Here's how the part is built. I have some questions about the finished solid (model axes, mm). A direction names the side the tool comes from. Round coordinates to 2 decimals unless told otherwise and drop trailing zeros. Write each loop counter-clockwise with the first axis right and the second up, starting at its lowest first coordinate (ties: lowest second). Pieces come first, ordered by that corner, then holes. Notation, with made-up numbers: (28, 58.25) - (83, 58.25) arc R5 ccw to (83, 64.25) - close; hole circle Ø1 at (-16.5, -35). An arc over 180 degrees is marked (long way). Write item = value, one per line. Start each with the question number.
Item 1: If we section it at A-A (z = 0): Please give me the cut outline in (x, y) (1 decimal).
Item 2: If I drill on line 1 along Y through (x, z) = (8, 0); line 2 along X through (y, z) = (12, -8.5) (3 decimals); line 3 along Y through (x, z) = (16.5, 7), over which ranges is the centre line in solid material (lowest first)? Write a range as [from, to].
Item 3: Which directions (+Z, -Z, +X, -X, +Y, -Y) give clear straight access to the entire face, cutting with the end or side of a thin tool? Please do faces 1 (the face through (13.148, 0.628, 14.274)), 2 (the face through (-3.175, -8, -8)).
Item 4: If we section it at C-C (x = 9.5): Please give me the cut outline in (y, z) (1 decimal), and give its area (3 significant figures).
Item 5: Thinking about a two-plate mould opening in Y: for faces 3 (the face through (29.845, -8, -8)), 4 (the face through (13.566, 8.406, -5.36)), 5 (the face through (-2.209, -10.626, 13.858)), which applies, pulls with the +Y half, pulls with the -Y half, needs draft (parallel to the pull), parting line crosses it, or undercut?
Item 6: For P1, Ø8, axis at x = 25, z = 8.5, coming from the -Y side; P2, Ø5, axis at x = 3.5, z = -11.5, coming from the +Y side; P3, Ø5, axis at x = 14.5, y = 7.5, coming from the -Z side; P4, Ø18, axis at y = 0, z = 0, coming from the -X side (3 decimals), each with a flat end and sliding along its axis, tell me the tip position at first contact or that it passes through.
```python
from build123d import *

# Parameters (mm, degrees)
SKETCH1_R            = 14.2875
SKETCH1_R_2          = 9.9695
BOSS_EXTRUDE1_DEPTH  = 26.67
SKETCH2_R            = 17.4625
SKETCH2_R_2          = 9.9695
BOSS_EXTRUDE2_DEPTH  = 3.175
FILLET1_R            = 1.27
FILLET1_OF_MIRROR1_R = 1.27


with BuildPart() as part:
    # Sketch1 → Boss-Extrude1 (new body)
    with BuildSketch(Plane(origin=(0, 0, 0), x_dir=(0, 0, -1), z_dir=(1, 0, 0))):
        Circle(SKETCH1_R)
        Circle(SKETCH1_R_2, mode=Mode.SUBTRACT)
    extrude(amount=BOSS_EXTRUDE1_DEPTH)

    # Sketch2 → Boss-Extrude2 (add)
    with BuildSketch(Plane(origin=(26.67, 0, 0), x_dir=(0, 0, -1), z_dir=(1, 0, 0))):
        Circle(SKETCH2_R)
        Circle(SKETCH2_R_2, mode=Mode.SUBTRACT)
    boss_extrude2 = extrude(amount=BOSS_EXTRUDE2_DEPTH)

    # Fillet1
    fillet1_edges = [part.edges().sort_by_distance(p)[0] for p in [
        (26.67, 0, 17.4625),
    ]]
    fillet(fillet1_edges, radius=FILLET1_R)

    # Mirror1: Boss-Extrude2 across plane
    add(boss_extrude2.mirror(Plane.ZY.offset(-13.335)))

    # Fillet1 of Mirror1
    fillet1_of_mirror1_edges = [part.edges().sort_by_distance(p)[0] for p in [
        (0, 0, 17.4625),
    ]]
    fillet(fillet1_of_mirror1_edges, radius=FILLET1_OF_MIRROR1_R)


solid = part.part
```
Reply:
q1.outline = (-3.2, -17.5) - (-1.3, -17.5) arc R1.3 ccw to (0, -16.2) - (0, -14.3) - (26.7, -14.3) - (26.7, -16.2) arc R1.3 ccw to (27.9, -17.5) - (29.8, -17.5) - (29.8, -10) - (-3.2, -10) - close; (-3.2, 10) - (29.8, 10) - (29.8, 17.5) - (27.9, 17.5) arc R1.3 ccw to (26.7, 16.2) - (26.7, 14.3) - (0, 14.3) - (0, 16.2) arc R1.3 ccw to (-1.3, 17.5) - (-3.2, 17.5) - close
q2.line_1 = [-14.29, -9.97], [9.97, 14.29]
q2.line_2 = [-3.175, 0], [26.67, 29.845]
q2.line_3 = [-12.46, -7.1], [7.1, 12.46]
q3.face_1 = none
q3.face_2 = +Z, -Z, -X, +Y, -Y
q4.outline = circle Ø28.6 at (0, 0); hole circle Ø19.9 at (0, 0)
q4.area = 329 mm2
q5.face_3 = needs draft
q5.face_4 = undercut
q5.face_5 = parting line crosses it
q6.P1 = -16.54
q6.P2 = 11.1
q6.P3 = -13.38
q6.P4 = through
